```python
from build123d import *

# Parameters (mm, degrees)
F0_W     = 304.8
F0_H     = 90.5500094
F0_W_2   = 11.5876832
F0_H_2   = 24
F0_R     = 3.175
F1_DEPTH = 3.175
F2_R     = 2.15265
F3_DEPTH = 3.175
F4_W     = 9.525
F4_H     = 9.525
F5_DEPTH = 3.175


with BuildPart() as f1:
    # F0 (on Top) → F1 (new body)
    with BuildSketch(Plane.XY):
        with Locations((152.4, -45.2750047)):
            Rectangle(F0_W, F0_H)
        with Locations((50.8, -75.3750094)):
            Rectangle(F0_W_2, F0_H_2, mode=Mode.SUBTRACT)
        with Locations((254, -75.3750094)):
            Rectangle(F0_W_2, F0_H_2, mode=Mode.SUBTRACT)
        with Locations((50.8, -15.175)):
            Rectangle(F0_W_2, F0_H_2, mode=Mode.SUBTRACT)
        with Locations((152.4, -45.2750047)):
            Circle(F0_R, mode=Mode.SUBTRACT)
        with Locations((254, -15.175)):
            Rectangle(F0_W_2, F0_H_2, mode=Mode.SUBTRACT)
    extrude(amount=F1_DEPTH)

    # F2 (on face) → F3 (cut, through all)
    with BuildSketch(Plane.XY.offset(3.175)):
        with Locations((4.7625, -14.2875)):
            Circle(F2_R)
        with Locations((4.7625, -76.2625094)):
            Circle(F2_R)
        with Locations((300.0375, -76.2625094)):
            Circle(F2_R)
        with Locations((300.0375, -14.2875)):
            Circle(F2_R)
    extrude(amount=-F3_DEPTH, mode=Mode.SUBTRACT)

    # F4 (on face) → F5 (cut, through all)
    with BuildSketch(Plane.XY.offset(3.175)):
        with Locations((300.0375, -4.7625)):
            Rectangle(F4_W, F4_H)
        with Locations((300.0375, -85.7875094)):
            Rectangle(F4_W, F4_H)
        with Locations((4.7625, -85.7875094)):
            Rectangle(F4_W, F4_H)
        with Locations((4.7625, -4.7625)):
            Rectangle(F4_W, F4_H)
    extrude(amount=-F5_DEPTH, mode=Mode.SUBTRACT)


solid = f1.part
```
Part model, mm, in its own coordinate system. Give positions to 0.01 mm unless a question says otherwise; leave off trailing zeros. Order: outer loops, then holes, each group sorted by start corner. A loop starts at its lowest first (then second) coordinate and runs counter-clockwise, first axis right, second up. Notation, with made-up numbers: M 56,15.5 L 89,15.5 A26 ccw 89,46.5 Z; hole C 38,-1.75 d5. An arc over 180 degrees is marked long. Use a Markdown table: item, result. Add a question column.
(1) Saw through at C-C, the plane z = 0.8. Give the number of separate pieces and of enclosed holes in the cut face, and give its area (3 significant figures).
(2) Drop a flat-ended pin along its axis: P1, Ø1, axis at x = 301, z = 2, coming from the +Y side (3 decimals). Give the stop position or say it passes through.
(3) Probe line 1 along X through (y, z) = (-14.5, 0.75); line 2 along X through (y, z) = (-73.5, 1.45); line 3 along X through (y, z) = (-6.5, 0.8) (3 decimals). List the from-to ranges inside material, lowest first. Write a range as [from, to].
(4) Saw through at A-A, the plane x = 152.4. Give the cut face in (y, z) (3 decimals).
(5) Mould opens along X. For faces 1 (the face through (155.333, -46.491, 1.565)), 2 (the face through (150, -35, 0)) say: +X half, -X half, draft (parallel to the pull), parting line (faces both ways), or undercut.
(6) Saw through at B-B, the plane y = -84. Give the cut face in (x, z) (3 decimals), and give its area (3 significant figures).
Answer key:
| question | item | result |
|---|---|---|
| 1 | separate pieces | 1 |
| 1 | enclosed holes | 9 |
| 1 | area | 26,000 mm^2 |
| 2 | P1 | y = -9.525 |
| 3 | line 1 | [0, 2.62], [6.9, 45.01], [56.59, 248.21], [259.79, 297.9], [302.18, 304.8] |
| 3 | line 2 | [0, 45.01], [56.59, 248.21], [259.79, 304.8] |
| 3 | line 3 | [9.525, 45.006], [56.594, 248.206], [259.794, 295.275] |
| 4 | outline | M -90.55,0 L -48.45,0 L -48.45,3.175 L -90.55,3.175 Z; M -42.1,0 L 0,0 L 0,3.175 L -42.1,3.175 Z |
| 5 | face 1 | undercut |
| 5 | face 2 | draft |
| 6 | outline | M 9.525,0 L 45.006,0 L 45.006,3.175 L 9.525,3.175 Z; M 56.594,0 L 248.206,0 L 248.206,3.175 L 56.594,3.175 Z; M 259.794,0 L 295.275,0 L 295.275,3.175 L 259.794,3.175 Z |
| 6 | area | 834 mm^2 |
